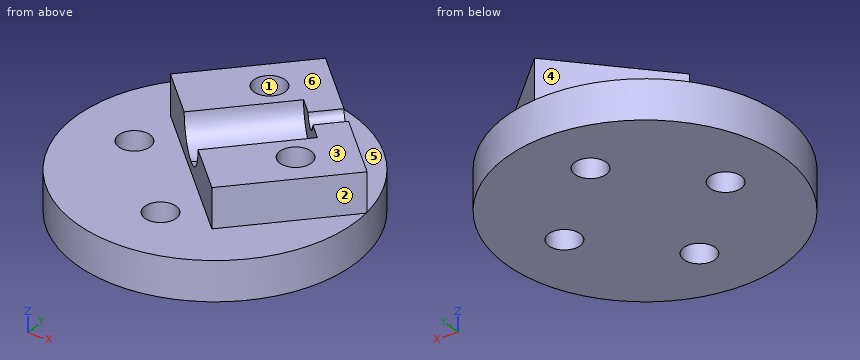
from build123d import *

# Parameters (mm, degrees)
SKETCH_1_R           = 14.149308539
SKETCH_1_R_2         = 1.6
EXTRUDE_1_DEPTH      = 4
EXTRUDE_2_DEPTH      = 11
EXTRUDE_2_DEPTH_BACK = 2
CUT_EXTRUDE_START    = -10
SKETCH_4_R           = 1.6
CUT_EXTRUDE_1_DEPTH  = 10
EXTRUDE_START        = -3
EXTRUDE_3_DEPTH      = 3


with BuildPart() as part:
    # 草图1 → 凸台-拉伸1 (new body)
    with BuildSketch(Plane.XY):
        Circle(SKETCH_1_R)
        with Locations((0, -8)):
            Circle(SKETCH_1_R_2, mode=Mode.SUBTRACT)
        with Locations((8, 0)):
            Circle(SKETCH_1_R_2, mode=Mode.SUBTRACT)
        with Locations((0, 8)):
            Circle(SKETCH_1_R_2, mode=Mode.SUBTRACT)
        with Locations((-8, 0)):
            Circle(SKETCH_1_R_2, mode=Mode.SUBTRACT)
    extrude(amount=EXTRUDE_1_DEPTH)

    # 草图3 → 凸台-拉伸2 (add, two sides: drawn at the far end of the back side and taken through both)
    with BuildSketch(Plane(origin=(0, 0, 0), x_dir=(0, 0, -1), z_dir=(0.7071067811865488, 0.7071067811865464, 0)).offset(-EXTRUDE_2_DEPTH_BACK)):
        with BuildLine():
            Line((-8, 9), (-8, 3))
            ThreePointArc((-8, 3), (-5.878679656, 2.121320344), (-5, 0))
            ThreePointArc((-5, 0), (-5.878679656, -2.121320344), (-8, -3))
            Line((-8, -3), (-8, -9))
            Line((-8, -9), (-4, -9))
            Line((-4, -9), (-4, 9))
            Line((-4, 9), (-8, 9))
        make_face()
    extrude(amount=EXTRUDE_2_DEPTH + EXTRUDE_2_DEPTH_BACK)

    # 草图4 → 切除-拉伸1 (cut)
    with BuildSketch(Plane.XY.offset(8).offset(CUT_EXTRUDE_START)):
        with Locations((8, 0)):
            Circle(SKETCH_4_R)
        with Locations((0, 8)):
            Circle(SKETCH_4_R)
    extrude(amount=CUT_EXTRUDE_1_DEPTH, mode=Mode.SUBTRACT)

    # 草图5 → 凸台-拉伸3 (add)
    with BuildSketch(Plane(origin=(7.778174593, 7.778174593, 0), x_dir=(0, 0, -1), z_dir=(0.7071067811865486, 0.7071067811865465, 0)).offset(EXTRUDE_START)):
        with BuildLine():
            Line((-8, -1), (-8, -3))
            ThreePointArc((-8, -3), (-5.878679656, -2.121320344), (-5, 0))
            ThreePointArc((-5, 0), (-5.878679656, 2.121320344), (-8, 3))
            Line((-8, 3), (-8, 1))
            ThreePointArc((-8, 1), (-7.292893219, 0.707106781), (-7, 0))
            ThreePointArc((-7, 0), (-7.292893219, -0.707106781), (-8, -1))
        make_face()
    extrude(amount=EXTRUDE_3_DEPTH)


solid = part.part
Geometry: final body of the model. Coordinates: model frame, mm. Face numbers are marked on the shaded views. A direction names the side the tool comes from. Coordinates: 2 decimals unless noted, no trailing zeros. Order: outer loops, then holes, each group sorted by start corner. A loop starts at its lowest first (then second) coordinate and runs counter-clockwise, first axis right, second up. Notation, with made-up numbers: (69.25, 87) - (88.25, 87) arc R9 cw to (88.25, 103) - close; hole circle Ø2 at (55.5, 66.5). An arc over 180 degrees is marked (long way). Use one line per item in the form item = value.
1) Ray query, L1, parallel to Z at x = -3.25, y = -10.75; L2, parallel to Z at x = -1, y = -1.25; L3, parallel to Y at x = 8, z = 3.5. Return the intervals inside material, ascending.
Solutions:
L1 = 0 to 4
L2 = 0 to 5.01
L3 = -11.67 to -1.6, 1.6 to 11.67
2) Section D-D (y = 0). State how many separate pieces and enclosed holes the cut face has, then the cut area to 3 significant figures.
Solutions:
separate_pieces = 3
enclosed_holes = 0
area = 119 mm^2
3) Pin query (flat end, axial travel): pin 1 (10 mm diameter, centred on x = 10.5, y = 8, fed in from +Z); pin 2 (1 mm diameter, centred on y = 6.5, z = 5.5, fed in from +X); pin 3 (1 mm diameter, centred on x = 8.5, z = 2, fed in from -Y); pin 4 (2 mm diameter, centred on x = 11, y = -7.5, fed in from +Z). Return the tip coordinate at first contact, or that it passes through.
Solutions:
pin_1 = 8
pin_2 = 9.56
pin_3 = -11.67
pin_4 = 4
4) Section C-C (z = 5.5). Return loops of the section in (x, y).
Solutions:
outline = (-7.78, 4.95) - (-2.59, -0.24) - (4.48, 6.83) - (6.83, 4.48) - (-0.24, -2.59) - (4.95, -7.78) - (14.14, 1.41) - (1.41, 14.14) - close; hole circle Ø3.2 at (0, 8); hole circle Ø3.2 at (8, 0)
5) Section A-A (z = 3). Return loops of the section in (x, y).
Solutions:
outline = circle Ø28.3 at (0, 0); hole circle Ø3.2 at (-8, 0); hole circle Ø3.2 at (0, -8); hole circle Ø3.2 at (0, 8); hole circle Ø3.2 at (8, 0)
6) Set-up query: the marked faces 4, 5 and 6. Return all of +Z, -Z, +X, -X, +Y, -Y with unobstructed straight access to the full face (end or side cutting, diameter ignored); none if empty.
Solutions:
face_4 = +Z, -X, +Y
face_5 = +Z, +X, +Y
face_6 = +Z, +X, -X, +Y, -Y
7) Mould query, pull axis X, two halves, no side actions, for the marked faces 1, 2 and 3. Classes: +X half, -X half, draft (parallel to the pull), parting line (faces both ways), or undercut.
Solutions:
face_1 = undercut
face_2 = +X half
face_3 = draft
8) Section B-B (x = 11.75). Return loops of the section in (y, z).
Solutions:
outline = (-7.88, 0) - (7.88, 0) - (7.88, 4) - (3.81, 4) - (3.81, 8) - (-0.98, 8) - (-0.98, 4) - (-7.88, 4) - close
